The model under review builds one solid part; all positions refer to its coordinate system, in mm. Face numbers are marked on the shaded views. A direction names the side the tool comes from. Round coordinates to 2 decimals unless told otherwise and drop trailing zeros. Loops run counter-clockwise (first coordinate to the right, second up) from the corner with the lowest first, then second, coordinate; pieces in that order, holes last. Notation, with made-up numbers: M -35,61.5 L 18,61.5 A35 cw 18,98.5 Z; hole C 11,62.25 d1. An arc over 180 degrees is marked long. Use a Markdown table: item, result. Add a question column.
```python
from build123d import *

# Parameters (mm, degrees)
PAD_DEPTH = 200


with BuildPart() as part:
    # Sketch → Pad (new body)
    with BuildSketch(Plane.XZ):
        Polygon((-38.415913, 63), (-38.415913, 51), (1.584087, 51), (1.584087, 0), (-38.415913, 0), (-38.415913, -12), (51.584087, -12), (51.584087, 0), (11.584087, 0), (11.584087, 51), (51.584087, 51), (51.584087, 63), align=None)
    extrude(amount=PAD_DEPTH)


solid = part.part
```
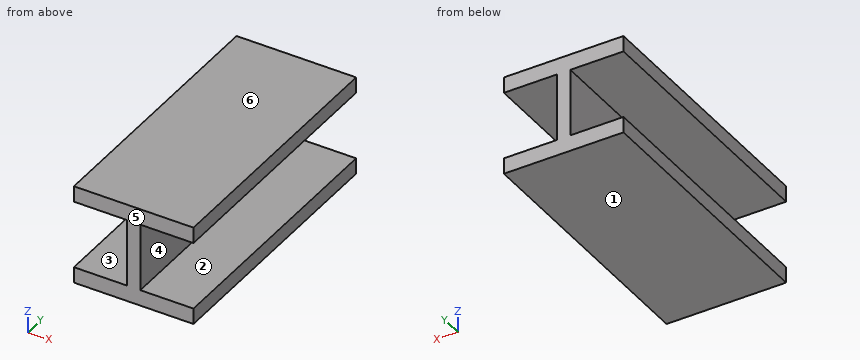
(1) For the marked faces 1, 2 and 3, list the 3-axis set-ups (+Z, -Z, +X, -X, +Y, -Y) from which the entire face can be reached by the end or side of a thin tool; tool diameter is ignored.
(2) Consider section B-B, the plane y = -27. Give the boundary of the cut face in (x, z).
(3) Insertion check: pin 1 Ø3 at (x, z) = (9.5, 33) entering from +Y; pin 2 Ø3 at (y, z) = (-24.5, 32.5) entering from +X. Each pin has a flat end and moves straight along its axis. Give the tip position at first contact, or say it passes through.
(4) Draft analysis for pull direction Z (two halves, no side actions). For the marked faces 4, 5 and 6, state which applies: released by +Z, released by -Z, zero draft, split by the parting line, or undercut.
(5) Consider section C-C, the plane z = 18. Give the boundary of the cut face in (x, y), then the cut area to 3 significant figures.
(6) To check wall thickness, follow probe 1 along Z at (x, y) = (47.5, -24.5); probe 2 along X at (y, z) = (-33, 39). State the ranges of each line that lie inside material, in increasing order.
(7) Consider section A-A, the plane x = -9.5. Give the boundary of the cut face in (y, z).
Found:
| question | item | result |
|---|---|---|
| 1 | face 1 | -Z, +X, -X, +Y, -Y |
| 1 | face 2 | +X, +Y, -Y |
| 1 | face 3 | -X, +Y, -Y |
| 2 | outline | M -38.42,-12 L 51.58,-12 L 51.58,0 L 11.58,0 L 11.58,51 L 51.58,51 L 51.58,63 L -38.42,63 L -38.42,51 L 1.58,51 L 1.58,0 L -38.42,0 Z |
| 3 | pin 1 | stops at y = 0 |
| 3 | pin 2 | stops at x = 11.58 |
| 4 | face 4 | undercut |
| 4 | face 5 | zero draft |
| 4 | face 6 | released by +Z |
| 5 | outline | M 1.58,-200 L 11.58,-200 L 11.58,0 L 1.58,0 Z |
| 5 | area | 2,000 mm^2 |
| 6 | probe 1 | z = -12 to 0, 51 to 63 |
| 6 | probe 2 | x = 1.58 to 11.58 |
| 7 | outline | M -200,-12 L 0,-12 L 0,0 L -200,0 Z; M -200,51 L 0,51 L 0,63 L -200,63 Z |
